from build123d import *

# Parameters (mm, degrees)
F1_DEPTH = 5
F3_D     = 5
F4_R     = 4.99999
F5_R     = 4
F7_DEPTH = 2


# Not quite as in the source:
# - a fillet or chamfer is up to 0.001 mm smaller than in the source, because OpenCascade refuses the exact size
# - a feature names something its author has since deleted; it is built from what else it names


with BuildPart() as f1:
    # F0 (on Top) → F1 (new body, symmetric)
    with BuildSketch(Plane.XY):
        Polygon((13, -45), (56, -45), (56, 45), (13, 45), (-5, 45), (-5, 25), (11, 25), (11, -25), (-5, -25), (-5, -45), align=None)
        with BuildLine():
            ThreePointArc((43, -27.5), (48, -32.5), (43, -37.5))
            Line((43, -37.5), (21, -37.5))
            ThreePointArc((21, -37.5), (16, -32.5), (21, -27.5))
            Line((21, -27.5), (43, -27.5))
        make_face(mode=Mode.SUBTRACT)
        with BuildLine():
            ThreePointArc((43, 37.5), (48, 32.5), (43, 27.5))
            Line((43, 27.5), (21, 27.5))
            ThreePointArc((21, 27.5), (16, 32.5), (21, 37.5))
            Line((21, 37.5), (43, 37.5))
        make_face(mode=Mode.SUBTRACT)
    extrude(amount=F1_DEPTH, both=True)

    # F3 (through all)
    with Locations(Plane.XZ.offset(45)):
        with Locations((0, 0)):
            Hole(F3_D / 2)

    # F4 (radius 5 in the source; OpenCascade refuses exactly that, so slightly less here)
    f4_edges = [f1.edges().sort_by_distance(p)[0] for p in [
        (-5, -35, 5),
        (-5, -35, -5),
        (-5, 35, 5),
        (-5, 35, -5),
    ]]
    fillet(f4_edges, radius=F4_R)

    # F5
    f5_edges = [f1.edges().sort_by_distance(p)[0] for p in [
        (11, 25, 0),
        (11, -25, 0),
    ]]
    fillet(f5_edges, radius=F5_R)

    # F6 (on face) → F7 (cut)
    with BuildSketch(Plane.XY.offset(5)):
        with BuildLine():
            ThreePointArc((46, 5), (41, 0), (46, -5))
            Line((46, -5), (56, -5))
            Line((56, -5), (56, 5))
            Line((56, 5), (46, 5))
        make_face()
    extrude(amount=-F7_DEPTH, mode=Mode.SUBTRACT)


solid = f1.part
Design review of the part built by this model. Coordinates are the model's own, in mm. A direction names the side the tool comes from. Round coordinates to 2 decimals unless told otherwise and drop trailing zeros. Loops run counter-clockwise (first coordinate to the right, second up) from the corner with the lowest first, then second, coordinate; pieces in that order, holes last. Notation, with made-up numbers: M 12,-25 L 50,-25 A23 cw 50,10 Z; hole C -37,-37 d7. An arc over 180 degrees is marked long. Answer as a JSON object with one key per item and string values.
Item 1: Clearance check with flat-ended pins moving along their axes: P1, Ø3, axis at y = -1.5, z = 2.5, coming from the -X side; P2, Ø5, axis at x = 50.5, y = 2, coming from the +Z side; P3, Ø3, axis at x = 0, z = 0, coming from the -Y side. State where each tip first meets the part, or that it passes through.
Answer sheet:
{"P1": "stops at x = 11", "P2": "stops at z = 3", "P3": "passes through"}
Item 2: Machinability: for faces 1 (the cylindrical face through (16, 32.4, 0.1)), 2 (the cylindrical face through (-3, -35, -4)), 3 (the flat face through (51, 5, 4)), 4 (the flat face through (11, 0, 0)), which of the approach directions +Z, -Z, +X, -X, +Y, -Y give a long, thin tool a straight path to every point of the face, cutting with its end or side? Answer none if there is none.
Answer sheet:
{"face 1": "+Z, -Z", "face 2": "-Z, -X, +Y, -Y", "face 3": "+Z, +X", "face 4": "+Z, -Z, -X"}
Item 3: We need section C-C on z = -1. Give the boundary of the cut face in (x, y), and give its area (3 significant figures).
Answer sheet:
{"outline": "M -4.9,-45 L -2.29,-45 L -2.29,-25 L -4.9,-25 Z; M -4.9,25 L -2.29,25 L -2.29,45 L -4.9,45 Z; M 2.29,-45 L 56,-45 L 56,45 L 2.29,45 L 2.29,25 L 7,25 A4 cw 11,21 L 11,-21 A4 cw 7,-25 L 2.29,-25 Z; hole M 21,-37.5 L 43,-37.5 A5 ccw 43,-27.5 L 21,-27.5 A5 ccw Z; hole M 21,27.5 L 43,27.5 A5 ccw 43,37.5 L 21,37.5 A5 ccw Z", "area": "3,910 mm^2"}
Item 4: We need section B-B on x = 29.5. Give the boundary of the cut face in (y, z).
Answer sheet:
{"outline": "M -45,-5 L -37.5,-5 L -37.5,5 L -45,5 Z; M -27.5,-5 L 27.5,-5 L 27.5,5 L -27.5,5 Z; M 37.5,-5 L 45,-5 L 45,5 L 37.5,5 Z"}
Item 5: Wall thickness on L1, parallel to Y at x = 30, z = 3.25; L2, parallel to Y at x = 5, z = -1.75; L3, parallel to Z at x = 0, y = -33.25: over which ranges is each line inside the solid? List them lowest first. Write a range as from..to.
Answer sheet:
{"L1": "y = -45..-37.5, -27.5..27.5, 37.5..45", "L2": "y = -45..-25, 25..45", "L3": "z = -5..-2.5, 2.5..5"}
Item 6: We need section D-D on x = 18. Give the boundary of the cut face in (y, z), and give its area (3 significant figures).
Answer sheet:
{"outline": "M -45,-5 L -36.5,-5 L -36.5,5 L -45,5 Z; M -28.5,-5 L 28.5,-5 L 28.5,5 L -28.5,5 Z; M 36.5,-5 L 45,-5 L 45,5 L 36.5,5 Z", "area": "740 mm^2"}
Item 7: The part is to be moulded in two halves that separate along X. For faces 5 (the cylindrical face through (0.54, 35.14, -2.44)), 6 (the cylindrical face through (-3, -35, 4)), 7 (the flat face through (56, -1, 0)), say which applies: pulls with the +X half, pulls with the -X half, needs draft (parallel to the pull), parting line crosses it, or undercut.
Answer sheet:
{"face 5": "undercut", "face 6": "pulls with the -X half", "face 7": "pulls with the +X half"}
Item 8: We need section A-A on y = -32.5. State how many separate pieces and enclosed holes the cut face has, and give its area (3 significant figures).
Answer sheet:
{"separate pieces": "2", "enclosed holes": "1", "area": "260 mm^2"}
